```python
from build123d import *

# Parameters (mm, degrees)
F0_R     = 4.9657
F1_DEPTH = 3.175
F2_R     = 12.7


with BuildPart() as f1:
    # F0 (on Front) → F1 (new body, symmetric)
    with BuildSketch(Plane.XZ):
        Polygon((-83.226920908, -83.226920908), (0, 0), (0, 4.1710244843), (0, 116.7433295739), (-141.598585695, -24.8552561211), align=None)
        with Locations((-88.8395809837, -50.6734924691)):
            Circle(F0_R, mode=Mode.SUBTRACT)
        with Locations((-119.1479453923, -20.3651280605)):
            Circle(F0_R, mode=Mode.SUBTRACT)
        Polygon((0, 4.1710244843), (0, 0), (83.226920908, -83.226920908), (141.598585695, -24.8552561211), (0, 116.7433295739), align=None)
        with Locations((88.8395809837, -50.6734924691)):
            Circle(F0_R, mode=Mode.SUBTRACT)
        with Locations((119.1479453923, -20.3651280605)):
            Circle(F0_R, mode=Mode.SUBTRACT)
    extrude(amount=F1_DEPTH, both=True)

    # F2
    f2_edges = [f1.edges().sort_by_distance(p)[0] for p in [
        (-141.598586, 0, -24.855256),
        (0, 0, 116.74333),
        (0, 0, 0),
        (83.226921, 0, -83.226921),
        (141.598586, 0, -24.855256),
        (-83.226921, 0, -83.226921),
    ]]
    fillet(f2_edges, radius=F2_R)


solid = f1.part
```
Design review of the part built by this model. Coordinates are the model's own, in mm. A direction names the side the tool comes from. Coordinates: 2 decimals unless noted, no trailing zeros. Write each loop counter-clockwise with the first axis right and the second up, starting at its lowest first coordinate (ties: lowest second). Pieces come first, ordered by that corner, then holes.
1) Add section C-C (x = 67). Write out the cut boundary in (y, z) (3 decimals).
2) Add section A-A (z = -42.5). Write out the cut boundary in (x, y) (3 decimals), plus the area to 3 significant figures.
3) Insertion check: pin 1 (2 mm diameter, centred on y = -2, z = 19, fed in from +X); pin 2 (1.5 mm diameter, centred on y = -1, z = -8.5, fed in from +X). Each pin has a flat end and moves straight along its axis. Give the tip position at first contact, or say it passes through.
4) Machinability: for faces 4 (the flat face through (41, 0, -41)), 5 (the flat face through (-112.696, -0.044, -53.758)), which of the approach directions +Z, -Z, +X, -X, +Y, -Y give a long, thin tool a straight path to every point of the face, cutting with its end or side? Answer none if there is none.
5) To check wall thickness, follow L1, parallel to X at y = 1.5, z = -70; L2, parallel to Z at x = -120.5, y = 0; L3, parallel to Z at x = -78.5, y = -1.75. State the ranges of each line that lie inside material, in increasing order.
6) Mouldability with a two-part tool opening along Z and no side actions: class faces 1 (the cylindrical face through (-124.11, 0.04, -20.15)), 2 (the flat face through (-2, -3.175, -3)), 3 (the cylindrical face through (-136.337, 0.044, -24.995)) as +Z half, -Z half, draft (parallel to the pull), parting line (faces both ways), or undercut.
7) Add section D-D (z = 8). Write out the cut boundary in (x, y) (3 decimals), plus the area to 3 significant figures.
8) Add section B-B (y = 1.25). Write out the cut boundary in (x, z) (1 decimal), plus the area to 3 significant figures.
Check result:
1. outline: (-3.175, -67) - (3.175, -67) - (3.175, 49.743) - (-3.175, 49.743) - close
2. outline: (-123.954, -3.175) - (-42.5, -3.175) - (-42.5, 3.175) - (-123.954, 3.175) - close; (42.5, -3.175) - (123.954, -3.175) - (123.954, 3.175) - (42.5, 3.175) - close
2. area: 1,030 mm2
3. pin 1: stops at x = 98.74
3. pin 2: stops at x = 125.99
4. face 4: -Z, +Y, -Y
4. face 5: -Z, -X, +Y, -Y
5. L1: x = -96.45 to -70, 70 to 96.45
5. L2: z = -45.95 to -25.14, -15.59 to -3.76
5. L3: z = -77.05 to 38.24
6. face 1: undercut
6. face 2: draft
6. face 3: parting line
7. outline: (-108.743, -3.175) - (108.743, -3.175) - (108.743, 3.175) - (-108.743, 3.175) - close
7. area: 1,380 mm2
8. outline: (-132.6, -33.8) - (-92.2, -74.2) arc R12.7 ccw to (-74.2, -74.2) - (-9, -9) arc R12.7 cw to (9, -9) - (74.2, -74.2) arc R12.7 ccw to (92.2, -74.2) - (132.6, -33.8) arc R12.7 ccw to (132.6, -15.9) - (9, 107.8) arc R12.7 ccw to (-9, 107.8) - (-132.6, -15.9) arc R12.7 ccw to start; hole circle Ø9.9 at (-119.1, -20.4); hole circle Ø9.9 at (-88.8, -50.7); hole circle Ø9.9 at (88.8, -50.7); hole circle Ø9.9 at (119.1, -20.4)
8. area: 25,800 mm2
